Source: three-view drawing plus pictorial views. Frame: mm from the lowest corner of the part. Give positions to 0.01 mm unless a question says otherwise; leave off trailing zeros. Order: outer loops, then holes, each group sorted by start corner. A loop starts at its lowest first (then second) coordinate and runs counter-clockwise, first axis right, second up. Notation, with made-up numbers: (67, 76.5) -> (109, 76.5) arc R24 ccw to (109, 90.5) -> close; hole circle Ø9 at (87, -27.5). An arc over 180 degrees is marked (long way). One line per question, with ' | ' between items.
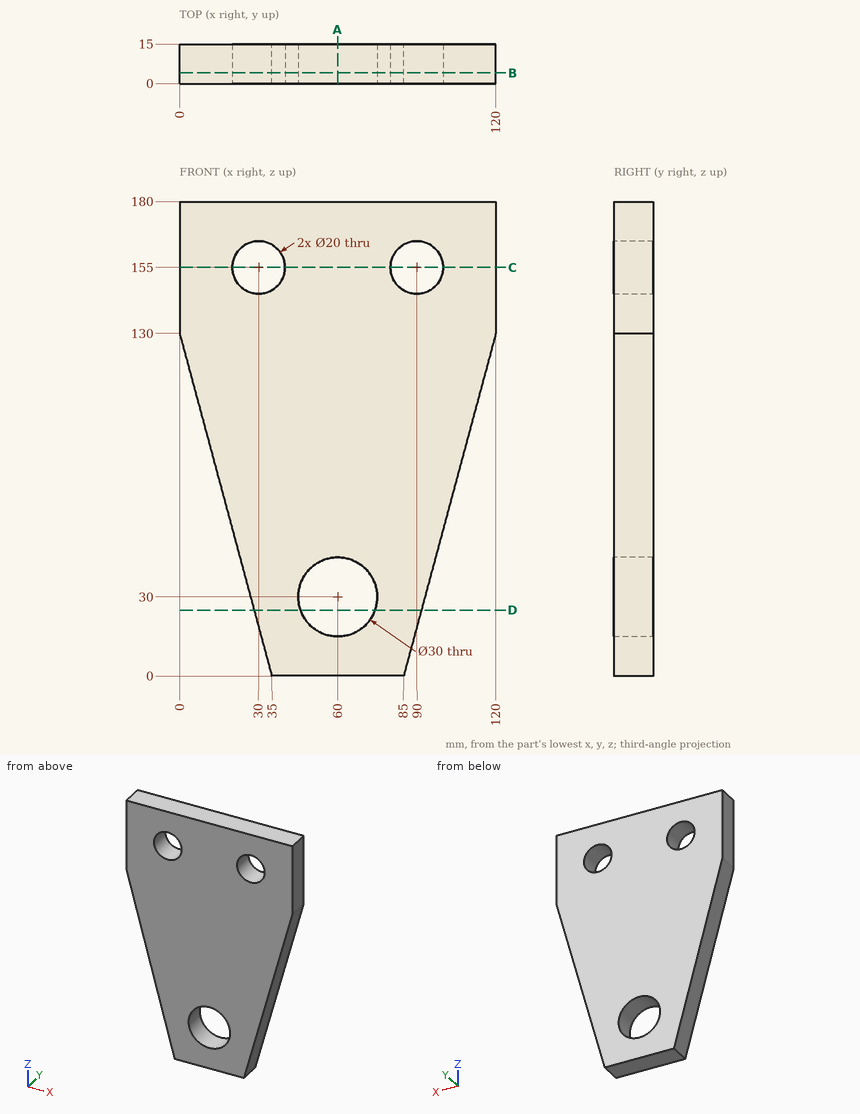
1) Section A-A on x = 60. Return loops of the section in (y, z).
Check result:
outline: (0, 0) -> (15, 0) -> (15, 15) -> (0, 15) -> close; (0, 45) -> (15, 45) -> (15, 180) -> (0, 180) -> close
2) Contact query for a flat-ended pin moving along its axis: pin 1 Ø16 at (x, z) = (90, 155) entering from -Y. Output: stop coordinate, or through.
Check result:
pin 1: passes through
3) Section B-B on y = 4. Return loops of the section in (x, z).
Check result:
outline: (0, 130) -> (35, 0) -> (85, 0) -> (120, 130) -> (120, 180) -> (0, 180) -> close; hole circle Ø20 at (30, 155); hole circle Ø30 at (60, 30); hole circle Ø20 at (90, 155)
4) Section D-D on z = 25. Return loops of the section in (x, y), plus the area to 3 significant figures.
Check result:
outline: (28.27, 0) -> (45.86, 0) -> (45.86, 15) -> (28.27, 15) -> close; (74.14, 0) -> (91.73, 0) -> (91.73, 15) -> (74.14, 15) -> close | area: 528 mm^2
5) Section C-C on z = 155. Return loops of the section in (x, y), plus the area to 3 significant figures.
Check result:
outline: (0, 0) -> (20, 0) -> (20, 15) -> (0, 15) -> close; (40, 0) -> (80, 0) -> (80, 15) -> (40, 15) -> close; (100, 0) -> (120, 0) -> (120, 15) -> (100, 15) -> close | area: 1,200 mm^2
6) Material intervals for probe 1 along X at (y, z) = (8.25, 155); probe 2 along X at (y, z) = (6.25, 159.5); probe 3 along Z at (x, y) = (81, 7), sorted ascending. Write a range as from..to.
Check result:
probe 1: x = 0..20, 40..80, 100..120 | probe 2: x = 0..21.07, 38.93..81.07, 98.93..120 | probe 3: z = 0..150.64, 159.36..180
